Design review of the part built by this model. Coordinates are the model's own, in mm. A direction names the side the tool comes from. Give positions to 0.01 mm unless a question says otherwise; leave off trailing zeros. Loops run counter-clockwise (first coordinate to the right, second up) from the corner with the lowest first, then second, coordinate; pieces in that order, holes last. Notation, with made-up numbers: (-37.5, 53.5) -> (-30.5, 53.5) arc R19 ccw to (-30.5, 75.5) -> close; hole circle Ø11 at (-3.75, -18). An arc over 180 degrees is marked (long way). Answer in a Markdown table with one row per item. Add a question column.
(1) Consider section C-C on x = -26.5. Write out the cut boundary in (y, z), then the cut area to 3 significant figures.
(2) For line 1 (X direction, y = 2, z = 22.75); line 2 (Y direction, x = 9.5, z = 23.5); line 3 (Z direction, x = 4, y = -5), list the stretches that pass through material, from the lowest coordinate up.
(3) Consider section D-D on x = -2. Write out the cut boundary in (y, z).
(4) For pin 1 (2 mm diameter, centred on x = 5.5, y = -24, fed in from +Z); pin 2 (10 mm diameter, centred on x = -1, z = 9, fed in from -Y); pin 3 (5 mm diameter, centred on x = -2.5, y = -1.5, fed in from +Z), all flat-tipped, find the tip position at first contact; note any pin that passes through.
(5) Draft analysis for pull direction X (two halves, no side actions). For faces 5 (the flat face through (13.507, -12, 12)), 6 (the flat face through (4.867, 10, 13)), 7 (the flat face through (-40, -5, 25)), state which applies: +X half, -X half, draft (parallel to the pull), parting line (faces both ways), or undercut.
(6) For faces 1 (the flat face through (-16, -34.407, 1)), 2 (the cylindrical face through (-33.54, 6.89, 2.99)), 3 (the flat face through (-5.893, 10, 13)), 4 (the flat face through (11.507, -13, 14)), list the 3-axis set-ups (+Z, -Z, +X, -X, +Y, -Y) from which the entire face can be reached by the end or side of a thin tool; tool diameter is ignored.
(7) Consider section A-A on z = 5.25. Write out the cut boundary in (x, y), then the cut area to 3 significant figures.
(8) Consider section B-B on y = -17. Write out the cut boundary in (x, z).
from build123d import *

# Parameters (mm, degrees)
SKETCH_W        = 55
SKETCH_H        = 45
PAD_DEPTH       = 25
SKETCH001_W     = 51
SKETCH001_H     = 47.679478
POCKET_DEPTH    = 23
SKETCH002_R     = 1
PAD001_DEPTH    = 2
SKETCH003_W     = 10.76
SKETCH003_H     = 25.903362
POCKET001_DEPTH = 5


with BuildPart() as part:
    # Sketch → Pad (new body)
    with BuildSketch(Plane.XY):
        with Locations((-13.992789, -11.907131)):
            Rectangle(SKETCH_W, SKETCH_H)
    extrude(amount=PAD_DEPTH)

    # Sketch001 → Pocket (cut)
    with BuildSketch(Plane.XY.offset(25)):
        with Locations((-13.992789, -15.24687)):
            Rectangle(SKETCH001_W, SKETCH001_H)
    extrude(amount=-POCKET_DEPTH, mode=Mode.SUBTRACT)

    # Sketch002 → Pad001 (new body)
    with BuildSketch(Plane.XY.offset(2)):
        with Locations((-34.492789, 6.592869)):
            Circle(SKETCH002_R)
        with Locations((5.507211, -23.907131)):
            Circle(SKETCH002_R)
    extrude(amount=PAD001_DEPTH)

    # Sketch003 → Pocket001 (cut)
    with BuildSketch(Plane.XZ.offset(-8.592869)):
        with Locations((-0.512789, 14.951681)):
            Rectangle(SKETCH003_W, SKETCH003_H)
    extrude(amount=-POCKET001_DEPTH, mode=Mode.SUBTRACT)


solid = part.part
Values follow:
| question | item | result |
|---|---|---|
| 1 | outline | (-34.41, 0) -> (10.59, 0) -> (10.59, 25) -> (8.59, 25) -> (8.59, 2) -> (-34.41, 2) -> close |
| 1 | area | 136 mm2 |
| 2 | line 1 | -41.49 to -39.49, 11.51 to 13.51 |
| 2 | line 2 | 8.59 to 10.59 |
| 2 | line 3 | 0 to 2 |
| 3 | outline | (-34.41, 0) -> (10.59, 0) -> (10.59, 2) -> (-34.41, 2) -> close |
| 4 | pin 1 | z = 4 |
| 4 | pin 2 | y = 8.59 |
| 4 | pin 3 | z = 2 |
| 5 | face 5 | +X half |
| 5 | face 6 | undercut |
| 5 | face 7 | draft |
| 6 | face 1 | +Z, -Z, +X, -X, -Y |
| 6 | face 2 | +Z |
| 6 | face 3 | +Z, +Y, -Y |
| 6 | face 4 | +Z, -Y |
| 7 | outline | (-41.49, -34.41) -> (-39.49, -34.41) -> (-39.49, 8.59) -> (-5.89, 8.59) -> (-5.89, 10.59) -> (-41.49, 10.59) -> close; (4.87, 8.59) -> (11.51, 8.59) -> (11.51, -34.41) -> (13.51, -34.41) -> (13.51, 10.59) -> (4.87, 10.59) -> close |
| 7 | area | 260 mm2 |
| 8 | outline | (-41.49, 0) -> (13.51, 0) -> (13.51, 25) -> (11.51, 25) -> (11.51, 2) -> (-39.49, 2) -> (-39.49, 25) -> (-41.49, 25) -> close |
